Autodesk Inventor part; units mm, degrees
ref_plane "shtrmnl_XY" through (0, 0, 0) normal (0, 1, 0) x (1, 0, 0)
ref_plane "shtrmnl_YZ" through (0, 0, 0) normal (1, 0, 0) x (0, 0, -1)
ref_plane "shtrmnl_ZX" through (0, 0, 0) normal (0, 0, -1) x (0, 1, 0)
sketch "Sketch_1" plane through (0, 0, 0) normal (0, 1, 0) x (-1, 0, 0)
  line L0 (4.7244, 6.35) -> (3.2385, 6.35)
  line L1 (3.2385, 6.35) -> (3.2385, 8.5471)
  arc A0 (3.2385, 8.5471) -> (1.8415, 8.5471) centre (2.54, 8.5471) ccw
  line L2 (1.8415, 8.5471) -> (1.8415, 6.35)
  line L3 (1.8415, 6.35) -> (-1.8415, 6.35)
  line L4 (-1.8415, 6.35) -> (-1.8415, 8.5471)
  arc A1 (-1.8415, 8.5471) -> (-3.2385, 8.5471) centre (-2.54, 8.5471) ccw
  line L5 (-3.2385, 8.5471) -> (-3.2385, 6.35)
  line L6 (-3.2385, 6.35) -> (-4.7244, 6.35)
  line L7 (-4.7244, 6.35) -> (-4.7244, -6.35)
  line L8 (-4.7244, -6.35) -> (4.7244, -6.35)
  line L9 (4.7244, -6.35) -> (4.7244, 6.35)
extrude "Extrusion1" add sketch "Sketch_1" along normal blind 0.4064
ref_plane "shtrmnl_XY" through (0, 0, 0) normal (0, 1, 0) x (1, 0, 0)
ref_plane "shtrmnl_YZ" through (0, 0, 0) normal (1, 0, 0) x (0, 0, -1)
ref_plane "shtrmnl_ZX" through (0, 0, 0) normal (0, 0, -1) x (0, 1, 0)
properties part number "M202830TX-switch"
Source: CAD feature listing. Evaluate the final solid. Frame: model axes, mm. Coordinates: 2 decimals unless noted, no trailing zeros. Loops run counter-clockwise (first coordinate to the right, second up) from the corner with the lowest first, then second, coordinate; pieces in that order, holes last. Notation, with made-up numbers: (81.25, 83.5) -> (108.25, 83.5) arc R10 cw to (108.25, 102.5) -> close; hole circle Ø1 at (85.25, 84). An arc over 180 degrees is marked (long way). Answer in a Markdown table with one row per item. Add a question column.
Q1. Section A-A on y = 0.15. Return the cut outline in (x, z), and give its area (3 significant figures).
Q2. Ray query, line 1 along Z through (x, y) = (0.25, 0.3); line 2 along Z through (x, y) = (-2.5, 0.1). Return the intervals inside material, ascending.
Q3. Pull-direction query (Y, two-part tool) for faces 1 (the face through (0, 0, 2)), 2 (the face through (0, 0.406, 2)); classes: pulls with the +Y half, pulls with the -Y half, needs draft (parallel to the pull), parting line crosses it, or undercut.
Q4. Contact query for a flat-ended pin moving along its axis: pin 1 Ø2 at (x, z) = (-2.5, 0.5) entering from -Y. Output: stop coordinate, or through.
Computed values:
| question | item | result |
|---|---|---|
| 1 | outline | (-4.72, -6.35) -> (4.72, -6.35) -> (4.72, 6.35) -> (3.24, 6.35) -> (3.24, 8.55) arc R0.7 ccw to (1.84, 8.55) -> (1.84, 6.35) -> (-1.84, 6.35) -> (-1.84, 8.55) arc R0.7 ccw to (-3.24, 8.55) -> (-3.24, 6.35) -> (-4.72, 6.35) -> close |
| 1 | area | 128 mm^2 |
| 2 | line 1 | z = -6.35 to 6.35 |
| 2 | line 2 | z = -6.35 to 9.24 |
| 3 | face 1 | pulls with the -Y half |
| 3 | face 2 | pulls with the +Y half |
| 4 | pin 1 | stops at y = 0 |
